Autodesk Inventor part; units mm, degrees
ref_plane "YZ Plane" through (0, 0, 0) normal (1, 0, 0) x (0, 1, 0)
ref_plane "XZ Plane" through (0, 0, 0) normal (0, 1, 0) x (-1, 0, 0)
ref_plane "XY Plane" through (0, 0, 0) normal (0, 0, 1) x (1, 0, 0)
sketch "Sketch1" plane through (0, 0, 0) normal (0, 1, 0) x (-1, 0, 0)
  circle A0 centre (0, 0) radius 3
  circle A1 centre (0, 0) radius 11
  dimension "d0" = 6
  dimension "d1" = 22
extrude "Extrusion1" add sketch "Sketch1" against normal blind 10 contours A0
sketch "Sketch2" plane through (0, 0, 0) normal (0, 1, 0) x (1, 0, 0)
  circle A0 centre (0, 0) radius 3
  circle A1 centre (0, 0) radius 11
  dimension "d4" = 6
  dimension "d5" = 22
extrude "Extrusion2" add sketch "Sketch2" along normal blind 5 contours A0 | A1
sketch "Sketch3" plane through (0, 5, 0) normal (0, 1, 0) x (1, 0, 0)
  circle A0 centre (0, 0) radius 1.5
  dimension "d8" = 3
extrude "Extrusion3" cut sketch "Sketch3" against normal up to next
sketch "Sketch4" plane through (0, 5, 0) normal (0, 1, 0) x (1, 0, 0)
  circle A0 centre (-6.878, -4.0857) radius 1
  circle A1 centre (4.0857, -6.878) radius 1
  circle A2 centre (6.878, 4.0857) radius 1
  circle A3 centre (-4.0857, 6.878) radius 1
  circle A4 centre (0, 0) radius 1.5
  dimension "d11" = 2
  dimension "d14" = 360
  dimension "d17" = 5.5
  dimension "d18" = 3
extrude "Extrusion4" cut sketch "Sketch4" against normal up to next contours A0 | A1 | A2 | A3
properties part number "axe_ax12" material "ABS Plastic"
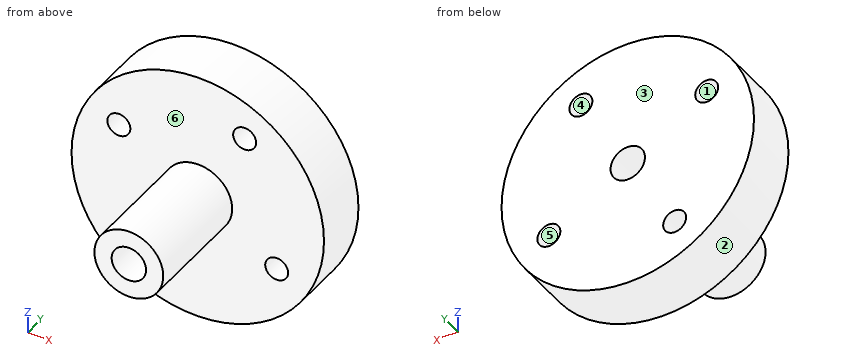
CAD build for the part. Positions are in the model's coordinates, mm. Face numbers are marked on the shaded views. A direction names the side the tool comes from. Give positions to 0.01 mm unless a question says otherwise; leave off trailing zeros. Write each loop counter-clockwise with the first axis right and the second up, starting at its lowest first coordinate (ties: lowest second). Pieces come first, ordered by that corner, then holes. Notation, with made-up numbers: (41, 78) - (63, 78) arc R30 cw to (63, 103) - close; hole circle Ø3 at (-10.5, -39). An arc over 180 degrees is marked (long way). Put each result on its own line as item: value.
(1) Saw through at D-D (z = 4.5). List the corners of the cut face in (x, y).
Working result:
outline: (-10.04, 0) - (-7.79, 0) - (-7.79, 5) - (-10.04, 5) - close; (-5.97, 0) - (10.04, 0) - (10.04, 5) - (-5.97, 5) - close
(2) Drop flat-ended pins along their axis: pin 1 Ø1.5 at (y, z) = (-4, 1.5) entering from -X; pin 2 Ø6 at (x, y) = (-5.5, 1) entering from -Z; pin 3 Ø4 at (x, y) = (-6.5, 2.5) entering from -Z; pin 4 Ø1.2 at (x, z) = (6.88, -4.09) entering from +Y. Give the stop position or say it passes through.
Working result:
pin 1: x = -2.9
pin 2: z = -10.71
pin 3: z = -10.04
pin 4: through
(3) Saw through at C-C (y = -2.75). List the corners of the cut face in (x, z), then the cut area to 3 significant figures.
Working result:
outline: circle Ø6 at (0, 0); hole circle Ø3 at (0, 0)
area: 21.2 mm^2
(4) Saw through at B-B (z = 0). List the corners of the cut face in (x, y), then the cut area to 3 significant figures.
Working result:
outline: (-11, 0) - (-3, 0) - (-3, -10) - (-1.5, -10) - (-1.5, 5) - (-11, 5) - close; (1.5, -10) - (3, -10) - (3, 0) - (11, 0) - (11, 5) - (1.5, 5) - close
area: 125 mm^2
(5) Wall check: L1, parallel to Z at x = 0, y = -1.5; L2, parallel to Y at x = 3.5, z = -6.25; L3, parallel to Z at x = 7.5, y = 1.25. Give the ranges that are in metal, low to high.
Working result:
L1: -3 to -1.5, 1.5 to 3
L2: 0 to 5
L3: -8.05 to -4.87, -3.3 to 8.05
(6) Pull direction Z, two halves, no side cores. Call the marked faces 1, 2, 3 and 4: released by +Z, released by -Z, zero draft, split by the parting line, or undercut.
Working result:
face 1: undercut
face 2: split by the parting line
face 3: zero draft
face 4: undercut
(7) Tool access for the marked faces 5 and 6: list every direction of +Z, -Z, +X, -X, +Y, -Y with a clear straight run to the whole face (end or side of a thin tool).
Working result:
face 5: +Y, -Y
face 6: -Y
(8) Saw through at A-A (x = 0). List the corners of the cut face in (y, z), then the cut area to 3 significant figures.
Working result:
outline: (-10, -3) - (0, -3) - (0, -11) - (5, -11) - (5, -1.5) - (-10, -1.5) - close; (-10, 1.5) - (5, 1.5) - (5, 11) - (0, 11) - (0, 3) - (-10, 3) - close
area: 125 mm^2
